Could you check a few things on this model? Use its own coordinates, in mm. A direction names the side the tool comes from. Give positions to 0.01 mm unless a question says otherwise; leave off trailing zeros. Write each loop counter-clockwise with the first axis right and the second up, starting at its lowest first coordinate (ties: lowest second). Pieces come first, ordered by that corner, then holes. Notation, with made-up numbers: M 41.25,-21.75 L 95.25,-21.75 A23 cw 95.25,-6.75 Z; hole C 55.5,-5 d11. An arc over 180 degrees is marked long. One line per item, written item: value.
Autodesk Inventor part; units mm, degrees
ref_plane "YZ Plane" through (0, 0, 0) normal (1, 0, 0) x (0, 1, 0)
ref_plane "XZ Plane" through (0, 0, 0) normal (0, 1, 0) x (-1, 0, 0)
ref_plane "XY Plane" through (0, 0, 0) normal (0, 0, 1) x (1, 0, 0)
sketch "Sketch1" plane through (0, 0, 0) normal (0, 1, 0) x (-1, 0, 0)
  circle A0 centre (0, 0) radius 40
  circle A1 centre (0, 0) radius 25
  dimension "d1" = 50
  dimension "d13" = 15
extrude "Extrusion1" add sketch "Sketch1" along normal blind 5
sketch "Sketch2" plane through (0, 5, 0) normal (0, 1, 0) x (1, 0, 0)
  circle A0 centre (-33, 0) radius 1.25
  circle A1 centre (0, 0) radius 25
  circle A2 centre (0, 0) radius 33 construction
  dimension "d4" = 2.5
  dimension "d12" = 8
extrude "Extrusion2" cut sketch "Sketch2" against normal blind 10 contours A0
pattern_circular "Circular Pattern1" count 6 over 360 about axis through (0, 0, 0) along (0, 1, 0) of "Extrusion2"
sketch "Sketch3" plane through (0, 5, 0) normal (0, 1, 0) x (1, 0, 0)
  line L0 (-85, -42.5) -> (85, -42.5)
  line L1 (85, -42.5) -> (85, 42.5)
  line L2 (85, 42.5) -> (-85, 42.5)
  line L3 (-85, 42.5) -> (-85, -42.5)
  line L4 (-85, -42.5) -> (85, 42.5) construction
  line L5 (85, -42.5) -> (-85, 42.5) construction
  line L6 (34.5, 15.5) -> (65.5, 15.5) construction
  line L7 (65.5, 15.5) -> (65.5, -15.5) construction
  line L8 (65.5, -15.5) -> (34.5, -15.5) construction
  line L9 (34.5, -15.5) -> (34.5, 15.5) construction
  line L10 (34.5, 15.5) -> (65.5, -15.5) construction
  line L11 (65.5, 15.5) -> (34.5, -15.5) construction
  circle A0 centre (34.5, 15.5) radius 1.5
  circle A1 centre (65.5, 15.5) radius 1.5
  circle A2 centre (65.5, -15.5) radius 1.5
  circle A3 centre (34.5, -15.5) radius 1.5
  line L12 (0, 0) -> (50, 0) construction
  circle A4 centre (0, 0) radius 40
  circle A5 centre (0, 0) radius 40
  line L13 (-50, 42.5) -> (-50, -42.5)
  circle A6 centre (50, 0) radius 12
  dimension "d14" = 85
  dimension "d15" = 170
  dimension "d16" = 31
  dimension "d17" = 31
  dimension "d18" = 3
  dimension "d19" = 3
  dimension "d20" = 3
  dimension "d21" = 3
  dimension "d22" = 50
  dimension "d23" = 35
  dimension "d26" = 24
extrude "Extrusion3" add sketch "Sketch3" against normal blind 5 contours L13 L2 L1 L0
sketch "Sketch4" plane through (0, 5, 0) normal (0, 1, 0) x (1, 0, 0)
  arc A0 (39.56, -5.9166) -> (39.56, 5.9166) centre (50, 0) ccw
  circle A1 centre (50, 0) radius 12
  point P0 (0, 0)
  point P1 (39.56, 5.9166)
  point P2 (39.56, -5.9166)
extrude "Extrusion4" cut sketch "Sketch4" against normal blind 5
sketch "Sketch5" plane through (0, 5, 0) normal (0, 1, 0) x (1, 0, 0)
  circle A0 centre (65.5, 15.5) radius 1.5
  circle A1 centre (65.5, 15.5) radius 1.5
  line L0 (34.5, -15.5) -> (65.5, -15.5)
  line L1 (65.5, -15.5) -> (65.5, 15.5)
  line L2 (65.5, 15.5) -> (34.5, 15.5)
  line L3 (34.5, 15.5) -> (34.5, -15.5)
  circle A2 centre (50, 0) radius 12
  line L4 (34.5, -15.5) -> (65.5, 15.5) construction
  line L5 (65.5, -15.5) -> (34.5, 15.5) construction
  circle A3 centre (34.5, 15.5) radius 1.5
  circle A4 centre (34.5, -15.5) radius 1.5
  point P0 (0, 0)
  dimension "d30" = 3
  dimension "d31" = 3
extrude "Extrusion5" cut sketch "Sketch5" against normal blind 5 contours A3 L3 L2 | L2 L3 A3 | A4 L3 L0 | L0 L3 A4
sketch "Sketch6" plane through (0, 5, 0) normal (0, 1, 0) x (1, 0, 0)
  line L0 (-65.5, -55) -> (97.5, -55)
  line L1 (97.5, -55) -> (97.5, 55)
  line L2 (97.5, 55) -> (-65.5, 55)
  line L3 (-65.5, 55) -> (-65.5, -55)
  line L4 (-65.5, -55) -> (97.5, 55) construction
  line L5 (97.5, -55) -> (-65.5, 55) construction
  line L6 (-65.5, 4) -> (-58.8, 4)
  line L7 (-58.8, 4) -> (-58.8, -55)
  line L8 (-58.8, -55) -> (-65.5, -55)
  line L9 (-65.5, -55) -> (-65.5, 4)
  line L10 (97.5, 55) -> (90.8, 55)
  line L11 (90.8, 55) -> (90.8, -4)
  line L12 (90.8, -4) -> (97.5, -4)
  line L13 (97.5, -4) -> (97.5, 55)
  line L14 (-50, -42.5) -> (-50, 42.5)
  line L15 (85, 42.5) -> (85, -42.5)
  line L16 (-50, 42.5) -> (85, 42.5)
  line L17 (85, 42.5) -> (85, -42.5)
  line L18 (85, -42.5) -> (-50, -42.5)
  line L19 (-50, -42.5) -> (-50, 42.5)
  point P0 (0, 0)
  point P1 (16, 0)
  dimension "d34" = 16
  dimension "d35" = 110
  dimension "d36" = 163
  dimension "d37" = 6.7
  dimension "d38" = 6.7
  dimension "d40" = 51
  dimension "d41" = 51
extrude "Extrusion6" add sketch "Sketch6" against normal blind 5 contours L7 L6 L3 L2 L11 L12 L1 L0
sketch "Sketch7" plane through (0, 5, 0) normal (0, 1, 0) x (1, 0, 0)
  line L0 (97.5, -49) -> (89.5, -49)
  line L1 (89.5, -49) -> (89.5, -40)
  line L2 (89.5, -40) -> (97.5, -40)
  line L3 (97.5, -40) -> (97.5, -49)
  line L4 (-58.8, -55) -> (97.5, -55)
  line L5 (97.5, -55) -> (97.5, -4)
  line L6 (97.5, -28) -> (93.5, -28)
  line L7 (93.5, -28) -> (93.5, -32)
  line L8 (93.5, -32) -> (97.5, -32)
  line L9 (97.5, -32) -> (97.5, -28)
  point P0 (0, 0)
  dimension "d44" = 6
  dimension "d45" = 9
  dimension "d46" = 8
  dimension "d47" = 8
  dimension "d48" = 4
  dimension "d49" = 4
extrude "Extrusion7" cut sketch "Sketch7" against normal blind 5
fillet "Fillet2" radius 2 2 edges at (97.5, 2.5, 28) (97.5, 2.5, 32)
fillet "Fillet3" radius 1 2 edges at (93.5, 2.5, 28) (93.5, 2.5, 32)
fillet "Fillet4" radius 1 2 edges at (97.5, 2.5, 49) (97.5, 2.5, 40)
fillet "Fillet5" radius 5 1 edges at (97.5, 2.5, 55)
fillet "Fillet6" radius 4 2 edges at (89.5, 2.5, 40) (89.5, 2.5, 49)
fillet "Fillet7" radius 5 2 edges at (97.5, 2.5, 4) (-65.5, 2.5, -4)
fillet "Fillet8" radius 10 3 edges at (-58.8, 2.5, 55) (90.8, 2.5, -55) (-65.5, 2.5, -55)
sketch "Sketch8" plane through (0, 5, 0) normal (0, 1, 0) x (1, 0, 0)
  circle A0 centre (-61.5, 8) radius 1.35
  circle A1 centre (93.5, -8) radius 1.35
  line L0 (-60.5, 4) -> (-58.8, 4)
  line L1 (-65.5, 45) -> (-65.5, 9)
  line L2 (92.5, -4) -> (90.8, -4)
  line L3 (97.5, -26) -> (97.5, -9)
  point P0 (0, 0)
  dimension "d59" = 4
  dimension "d60" = 4
  dimension "d61" = 2.7
  dimension "d62" = 4
  dimension "d63" = 4
  dimension "d64" = 2.7
extrude "Extrusion8" cut sketch "Sketch8" against normal blind 5
sketch "Sketch9" plane through (0, 5, 0) normal (0, 1, 0) x (1, 0, 0)
  line L0 (-48, 44) -> (76, 44)
  line L1 (76, 44) -> (76, -39)
  line L2 (76, -39) -> (-48, -39)
  line L3 (-48, -39) -> (-48, 44)
  point P0 (0, 0)
extrude "Extrusion9" add sketch "Sketch9" against normal blind 5
sketch "Sketch10" plane through (0, 5, 0) normal (0, 1, 0) x (1, 0, 0)
  circle A0 centre (16, 0) radius 40
  line L0 (-58.8, 4) -> (-58.8, -45)
  point P0 (0, 0)
  dimension "d69" = 80
  dimension "d70" = 74.8
extrude "Extrusion10" cut sketch "Sketch10" against normal blind 5
sketch "Sketch11" plane through (0, 5, 0) normal (0, 1, 0) x (1, 0, 0)
  line L0 (-44, -30) -> (76, -30) construction
  line L1 (76, -30) -> (76, 30) construction
  line L2 (76, 30) -> (-44, 30) construction
  line L3 (-44, 30) -> (-44, -30) construction
  circle A0 centre (16, 0) radius 40 construction
  line L4 (-44, -30) -> (76, 30) construction
  line L5 (76, -30) -> (-44, 30) construction
  circle A1 centre (76, 30) radius 1.5
  circle A2 centre (-44, 30) radius 1.5
  circle A3 centre (-44, -30) radius 1.5
  circle A4 centre (76, -30) radius 1.5
  point P0 (0, 0)
  dimension "d73" = 60
  dimension "d74" = 120
  dimension "d75" = 3
  dimension "d76" = 3
  dimension "d77" = 3
  dimension "d78" = 3
extrude "Extrusion11" cut sketch "Sketch11" against normal blind 5
sketch "Sketch12" plane through (0, 5, 0) normal (0, 1, 0) x (1, 0, 0)
  line L0 (-160, 70) -> (160, 70)
  line L1 (160, 70) -> (160, -70)
  line L2 (160, -70) -> (-160, -70)
  line L3 (-160, -70) -> (-160, 70)
  line L4 (-160, 70) -> (160, -70) construction
  line L5 (160, 70) -> (-160, -70) construction
  point P0 (0, 0)
extrude "Extrusion12" cut sketch "Sketch12" against normal blind 3
properties part number "Microscope lid"
1) If we section it at C-C, the plane y = 1.6: Give the number of separate pieces and of enclosed holes in the cut face, then the cut area to 3 significant figures.
Outcome:
separate pieces: 1
enclosed holes: 7
area: 11,900 mm^2
2) Please list where these lines run through material, in increasing order: L1, parallel to Z at x = 76, y = 0.5; L2, parallel to Z at x = 16, y = 0.45; L3, parallel to X at y = 1.3, z = 30. Write a range as from..to.
Outcome:
L1: z = -55..-31.5, -28.5..28.5, 31.5..55
L2: z = -55..-40, 40..55
L3: x = -58.8..-45.5, -42.5..-10.46, 42.46..74.5, 77.5..93.5
3) On a 3-axis mill with a long thin cutter (end or side, diameter ignored), from which of +Z, -Z, +X, -X, +Y, -Y can I reach the whole of each face in a straight line? I mean faces 4 (the face through (90.703, 0.986, 47.859)), 5 (the face through (-55.79, 0.99, 52.15)). Say none if no direction works.
Outcome:
face 4: +X, +Y, -Y
face 5: +Z, -X, +Y, -Y
4) If we section it at A-A, the plane z = 0: Write out the boundary of the cut face in (x, y), then the cut area to 3 significant figures.
Outcome:
outline: M -58.8,0 L -24,0 L -24,2 L -58.8,2 Z; M 56,0 L 90.8,0 L 90.8,2 L 56,2 Z
area: 139 mm^2
5) If we section it at B-B, the plane x = 16: Write out the boundary of the cut face in (y, z), then the cut area to 3 significant figures.
Outcome:
outline: M 0,-55 L 2,-55 L 2,-40 L 0,-40 Z; M 0,40 L 2,40 L 2,55 L 0,55 Z
area: 60.0 mm^2
6) I'm going to push flat-ended pins straight in: pin 1 (8 mm diameter, centred on x = -8.5, z = 28.5, fed in from +Y); pin 2 (0.5 mm diameter, centred on x = 95, y = 1, fed in from -Z); pin 3 (0.5 mm diameter, centred on x = 92, y = 0.5, fed in from -Z); pin 4 (1 mm diameter, centred on y = 1.5, z = -19.5, fed in from +X). Where does each tip first touch, or does it pass through?
Outcome:
pin 1: stops at y = 2
pin 2: stops at z = 4.53
pin 3: stops at z = 4
pin 4: stops at x = 90.8
7) If we section it at D-D, the plane z = 47: Write out the boundary of the cut face in (x, y), then the cut area to 3 significant figures.
Outcome:
outline: M -58.6,0 L 90.04,0 L 90.04,2 L -58.6,2 Z
area: 297 mm^2
8) We'd pull the mould along Z, two halves only. Please class faces 1 (the face through (87.79, 0.99, -52.15)), 2 (the face through (-45.5, 1.01, -30.07)), 3 (the face through (96.07, 0.99, 53.5)): pulls with the +Z half, pulls with the -Z half, needs draft (parallel to the pull), parting line crosses it, or undercut.
Outcome:
face 1: pulls with the -Z half
face 2: undercut
face 3: pulls with the +Z half
